Can you work these out from the model? Positions are in its coordinate system, mm. A direction names the side the tool comes from. Round coordinates to 2 decimals unless told otherwise and drop trailing zeros. Loops run counter-clockwise (first coordinate to the right, second up) from the corner with the lowest first, then second, coordinate; pieces in that order, holes last.
from build123d import *

# Parameters (mm, degrees)
F0_W     = 1900
F0_H     = 30
F1_DEPTH = 690
F2_DEPTH = 1010
F0_H_2   = 950
F3_DEPTH = 25
F4_DEPTH = 790
F6_DEPTH = 1010
F5_W     = 600
F5_H     = 390
F7_DEPTH = 30


with BuildPart() as f1:
    # F0 (on Top) → F1 (new body)
    with BuildSketch(Plane.XY):
        with Locations((-1000, 995)):
            Rectangle(F0_W, F0_H)
        with Locations((-1000, 15)):
            Rectangle(F0_W, F0_H)
        Polygon((-1950, 1010), (-2000, 1010), (-2000, 0), (-1950, 0), (-1950, 30), (-1950, 980), align=None)
        Polygon((0, 1010), (-50, 1010), (-50, 980), (-50, 30), (-50, 0), (0, 0), align=None)
    extrude(amount=F1_DEPTH)

    # F0 (on Top) → F2 (join)
    with BuildSketch(Plane.XY):
        Polygon((-1950, 1010), (-2000, 1010), (-2000, 0), (-1950, 0), (-1950, 30), (-1950, 980), align=None)
    extrude(amount=F2_DEPTH)

    # F0 (on Top) → F3 (join)
    with BuildSketch(Plane.XY):
        with Locations((-1000, 505)):
            Rectangle(F0_W, F0_H_2)
    extrude(amount=F3_DEPTH)

    # F0 (on Top) → F4 (join)
    with BuildSketch(Plane.XY):
        Polygon((0, 1010), (-50, 1010), (-50, 980), (-50, 30), (-50, 0), (0, 0), align=None)
    extrude(amount=F4_DEPTH)

    # F5 (on face) → F6 (cut)
    with BuildSketch(Plane.XZ):
        with BuildLine():
            Line((-1950, 0), (-750, 0))
            ThreePointArc((-750, 0), (-767.573593, 42.426407), (-810, 60))
            Line((-810, 60), (-1890, 60))
            ThreePointArc((-1890, 60), (-1932.426407, 42.426407), (-1950, 0))
        make_face()
        with BuildLine():
            Line((-650, 0), (-50, 0))
            ThreePointArc((-50, 0), (-67.573593, 42.426407), (-110, 60))
            Line((-110, 60), (-590, 60))
            ThreePointArc((-590, 60), (-632.426407, 42.426407), (-650, 0))
        make_face()
    extrude(amount=-F6_DEPTH, mode=Mode.SUBTRACT)

    # F5 (on face) → F7 (cut)
    with BuildSketch(Plane.XZ):
        Polygon((-1439.458966, 490), (-1950, 490), (-1950, 100), (-1439.458966, 100), (-750, 100), (-750, 490), align=None)
        with Locations((-350, 295)):
            Rectangle(F5_W, F5_H)
    extrude(amount=-F7_DEPTH, mode=Mode.SUBTRACT)


solid = f1.part
(1) If we section it at A-A, the plane z = 219: List the corners of the cut face in (x, y) for me.
Worked answers:
outline: (-2000, 0) - (-1950, 0) - (-1950, 980) - (-50, 980) - (-50, 0) - (0, 0) - (0, 1010) - (-2000, 1010) - close; (-750, 0) - (-650, 0) - (-650, 30) - (-750, 30) - close
(2) If we section it at C-C, the plane x = -1206.5: List the corners of the cut face in (y, z) for me.
Worked answers:
outline: (0, 60) - (30, 60) - (30, 100) - (0, 100) - close; (0, 490) - (30, 490) - (30, 690) - (0, 690) - close; (980, 60) - (1010, 60) - (1010, 690) - (980, 690) - close
(3) For faces 1 (the flat face through (-701, 512, 25)), 2 (the flat face through (-1975, 512, 1010)), 3 (the cylindrical face through (-752.977, 502.643, 18.664)), which set-ups out of +Z, -Z, +X, -X, +Y, -Y let a thin tool reach every point of the face, with its end or its side?
Worked answers:
face 1: +Z
face 2: +Z, +X, -X, +Y, -Y
face 3: -Z, +Y, -Y
(4) If we section it at B-B, the plane y = 605: List the corners of the cut face in (x, z) for me.
Worked answers:
outline: (-2000, 0) - (-1950, 0) arc R60 cw to (-1944.54, 25) - (-1950, 25) - (-1950, 1010) - (-2000, 1010) - close; (-755.46, 25) arc R60 cw to (-750, 0) - (-650, 0) arc R60 cw to (-644.54, 25) - close; (-55.46, 25) arc R60 cw to (-50, 0) - (0, 0) - (0, 790) - (-50, 790) - (-50, 25) - close
(5) If I drill on line 1 (X direction, y = 230, z = 655.5); line 2 (Y direction, x = -1636, z = 660); line 3 (Y direction, x = -887.5, z = 228), over which ranges is the centre line in solid material (lowest first)?
Worked answers:
line 1: x = -2000 to -1950, -50 to 0
line 2: y = 0 to 30, 980 to 1010
line 3: y = 980 to 1010
(6) If we section it at D-D, the plane x = -686: List the corners of the cut face in (y, z) for me.
Worked answers:
outline: (0, 0) - (1010, 0) - (1010, 690) - (980, 690) - (980, 25) - (30, 25) - (30, 690) - (0, 690) - close
(7) Will these pins go through, and if not, where does the flat tip stop? P1, Ø15, axis at x = -276, y = 12.5, coming from the +Z side; P2, Ø9, axis at x = -247.5, y = 22, coming from the -Z side; P3, Ø1.6, axis at x = -53.5, y = 309.5, coming from the +Z side.
Worked answers:
P1: stops at z = 690
P2: stops at z = 60
P3: stops at z = 25
(8) If we mould it in two halves opening along Y, with no side actions, what happens to faces 4 (the flat face through (-50, 512, 402)), 5 (the flat face through (-25, 512, 790)), 6 (the flat face through (-1005, 0, 503)), 7 (the flat face through (-1013, 980, 427))? For each: released by +Y, released by -Y, zero draft, split by the parting line, or undercut.
Worked answers:
face 4: undercut
face 5: zero draft
face 6: released by -Y
face 7: undercut
